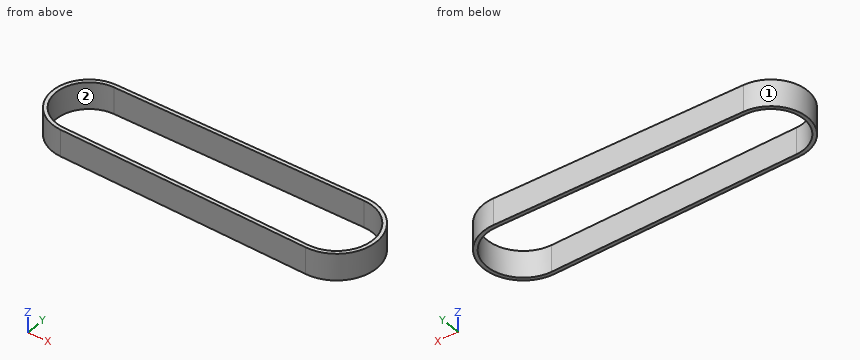
Autodesk Inventor part; units mm, degrees
ref_plane "Cross Section Plane" through (-0.2073, -15.1581, 0) normal (0.9999, -0.0137, 0) x (0, 0, 1)
ref_plane "Work Plane2" through (0, 0, 0) normal (0.309, 0.9511, 0) x (0, 0, 1)
ref_plane "Work Plane3" through (110.867, 0, 0) normal (-0.979, 0.2038, 0) x (0, 0, 1)
sketch "Sketch Path" plane through (0, 0, 0) normal (0, 0, 1) x (1, 0, 0)
  arc A0 (-0.2073, 15.1581) -> (-0.2073, -15.1581) centre (0, 0) ccw
  arc A1 (110.639, -16.6739) -> (110.639, 16.6739) centre (110.867, 0) ccw
  line L0 (110.639, -16.6739) -> (-0.2073, -15.1581)
  line L1 (-0.2073, 15.1581) -> (110.639, 16.6739)
ref_plane "Cross Section Plane" through (-0.2073, -15.1581, 0) normal (0.9999, -0.0137, 0) x (0, 0, 1)
ref_plane "Work Plane2" through (0, 0, 0) normal (0.309, 0.9511, 0) x (0, 0, 1)
ref_plane "Work Plane3" through (110.867, 0, 0) normal (-0.979, 0.2038, 0) x (0, 0, 1)
sketch "Cross Section" plane through (-0.2073, -15.1581, 0) normal (0.9999, -0.0137, 0) x (0, 0, 1)
  line L0 (-6, 1.27) -> (6, 1.27)
  line L1 (6, 1.27) -> (6, -0.381)
  line L2 (6, -0.381) -> (-6, -0.381)
  line L3 (-6, -0.381) -> (-6, 1.27)
  line L4 (-6, 0) -> (6, 0) construction
  point P0 (0, 0)
  point P1 (0, 0)
  dimension "d0" = 12
  dimension "d4" = 0.381
  dimension "d5" = 1.27
sweep "Belt" add profiles "Cross Section" path "Sketch Path"
equation "\"d4\" = da_a"
equation "\"d5\" = da_a2"
equation "\"da_B\" = 19.05"
equation "\"da_pb\" = 9.525"
equation "\"da_L\" = 321.76723"
equation "\"da_a\" = 0.381"
equation "\"da_S\" = 4.6482"
equation "\"da_Beta\" = 20deg"
equation "\"da_Ht\" = 1.905"
equation "\"da_H\" = 3.556"
equation "\"da_a2\" = 1.27"
properties part number "Synchronous Belt" material "Rubber"
Part model, mm, in its own coordinate system. Face numbers are marked on the shaded views. Give positions to 0.01 mm unless a question says otherwise; leave off trailing zeros. Order: outer loops, then holes, each group sorted by start corner. A loop starts at its lowest first (then second) coordinate and runs counter-clockwise, first axis right, second up. Notation, with made-up numbers: (13, 40) - (42, 40) arc R18 ccw to (42, 57) - close; hole circle Ø2 at (22, -38). An arc over 180 degrees is marked (long way). One line per question, with ' | ' between items.
1. Drill centre lines: probe 1 along X at (y, z) = (0.5, 3.5); probe 2 along X at (y, z) = (6.5, -5); probe 3 along Y at (x, z) = (29.5, 2). Where is each one in solid material? Low to high.
Filled in:
probe 1: -16.42 to -14.77, 127.15 to 128.81 | probe 2: -15.09 to -13.27, 125.81 to 127.59 | probe 3: -16.83 to -15.18, 15.18 to 16.83
2. Band-saw the part on C-C on x = 42.5. List the corners of the cut face in (y, z).
Filled in:
outline: (-17.01, -6) - (-15.36, -6) - (-15.36, 6) - (-17.01, 6) - close; (15.36, -6) - (17.01, -6) - (17.01, 6) - (15.36, 6) - close
3. Pull direction X, two halves, no side cores. Call the marked faces 1 and 2: +X half, -X half, draft (parallel to the pull), parting line (faces both ways), or undercut.
Filled in:
face 1: -X half | face 2: undercut
4. Drop flat-ended pins along their axis: P1, Ø2, axis at x = 31, z = 3, coming from the -Y side; P2, Ø6, axis at y = 11, z = 0, coming from the +X side; P3, Ø4, axis at x = 37.5, z = -4, coming from the -Y side. Give the stop position or say it passes through.
Filled in:
P1: y = -16.87 | P2: x = 126.93 | P3: y = -16.97
5. Band-saw the part on B-B on y = 0. List the corners of the cut face in (x, z).
Filled in:
outline: (-16.43, -6) - (-14.78, -6) - (-14.78, 6) - (-16.43, 6) - close; (127.16, -6) - (128.81, -6) - (128.81, 6) - (127.16, 6) - close
